```python
from build123d import *

# Parameters (mm, degrees)
BOSS_EXTRUDE1_DEPTH     = 60
SKETCH2_W               = 20
SKETCH2_H               = 25
CUT_EXTRUDE1_DEPTH      = 15
CUT_EXTRUDE2_DEPTH      = 137.47344064
CUT_EXTRUDE2_DEPTH_BACK = 137.47344064
SKETCH3_R               = 5


with BuildPart() as part:
    # Sketch1 → Boss-Extrude1 (new body)
    with BuildSketch(Plane.XY):
        Polygon((0, 0), (120, 0), (120, 43), (100, 43), (100, 15), (35, 15), (35, 25), (10, 25), (0, 20.336923418), align=None)
    extrude(amount=BOSS_EXTRUDE1_DEPTH)

    # Sketch2 → Cut-Extrude1 (cut)
    with BuildSketch(Plane(origin=(0, 43, 0), x_dir=(1, 0, 0), z_dir=(0, 1, 0))):
        with Locations((110, -30)):
            Rectangle(SKETCH2_W, SKETCH2_H)
    extrude(amount=-CUT_EXTRUDE1_DEPTH, mode=Mode.SUBTRACT)

    # Sketch3 → Cut-Extrude2 (cut, two sides: drawn at the far end of the back side and taken through both)
    with BuildSketch(Plane(origin=(0, 25, 0), x_dir=(1, 0, 0), z_dir=(0, 1, 0)).offset(-CUT_EXTRUDE2_DEPTH_BACK)):
        with Locations(Location((22.5, -40, 0), (0, 0, 180))):
            Circle(SKETCH3_R)
        with Locations(Location((22.5, -20, 0), (0, 0, 180))):
            Circle(SKETCH3_R)
    extrude(amount=CUT_EXTRUDE2_DEPTH + CUT_EXTRUDE2_DEPTH_BACK, mode=Mode.SUBTRACT)


solid = part.part
```
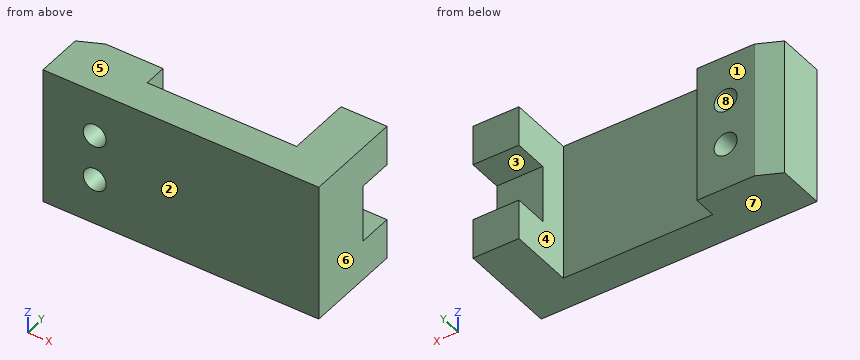
The listing builds one solid part. Answer for the finished solid, in the listing's coordinates (mm). Face numbers are marked on the shaded views. A direction names the side the tool comes from. Round coordinates to 2 decimals unless told otherwise and drop trailing zeros. Loops run counter-clockwise (first coordinate to the right, second up) from the corner with the lowest first, then second, coordinate; pieces in that order, holes last.
Q1. Section D-D, the plane y = 33.5 is taken. Determine the outline of the cut face in (x, z).
Q2. For a pull along Z with two mould halves and no side action, classify the marked faces 5, 6, 7 and 8 as released by +Z, released by -Z, zero draft, split by the parting line, or undercut.
Q3. Find the intervals of material crossed by line 1 (Z direction, x = 22.5, y = 19.5); line 2 (X direction, y = 16.5, z = 20); line 3 (X direction, y = 19, z = 56), in increasing order.
Q4. Which of the six approach directions +Z, -Z, +X, -X, +Y, -Y give full straight-line access (tool end or side, diameter ignored) to the marked faces 1, 2, 3 and 4?
Q5. Section C-C, the plane z = 20 is taken. Determine the outline of the cut face in (x, y), then the cut area to 3 significant figures.
Q6. Given pin 1 Ø2 at (x, z) = (25, 36.5) entering from -Y; pin 2 Ø10 at (x, z) = (105.5, 28) entering from +Y; pin 3 Ø8.5 at (y, z) = (31, 26) entering from -X; pin 4 Ø12 at (x, z) = (55.5, 9.5) entering from +Y, each flat-ended and moving along its own axis, determine where each tip first touches the part or whether it passes through.
Q7. Section A-A, the plane x = 22.5 is taken. Determine the outline of the cut face in (y, z).
Q8. Section B-B, the plane y = 17 is taken. Determine the outline of the cut face in (x, z), then the cut area to 3 significant figures.
Completed:
1. outline: (100, 0) - (120, 0) - (120, 17.5) - (100, 17.5) - close; (100, 42.5) - (120, 42.5) - (120, 60) - (100, 60) - close
2. face 5: released by +Z
2. face 6: zero draft
2. face 7: released by -Z
2. face 8: undercut
3. line 1: z = 0 to 15, 25 to 35, 45 to 60
3. line 2: x = 0 to 17.5, 27.5 to 35, 100 to 120
3. line 3: x = 0 to 35, 100 to 120
4. face 1: +Z, -Z, -X, +Y
4. face 2: +Z, -Z, +X, -X, -Y
4. face 3: +X, -X, +Y
4. face 4: +Z, -Z, +Y
5. outline: (0, 0) - (17.5, 0) - (17.5, 25) - (10, 25) - (0, 20.34) - close; (27.5, 0) - (120, 0) - (120, 28) - (100, 28) - (100, 15) - (35, 15) - (35, 25) - (27.5, 25) - close
5. area: 2,140 mm2
6. pin 1: stops at y = 0
6. pin 2: stops at y = 28
6. pin 3: stops at x = 100
6. pin 4: stops at y = 15
7. outline: (0, 0) - (25, 0) - (25, 15) - (0, 15) - close; (0, 25) - (25, 25) - (25, 35) - (0, 35) - close; (0, 45) - (25, 45) - (25, 60) - (0, 60) - close
8. outline: (0, 0) - (35, 0) - (35, 60) - (0, 60) - close; (100, 0) - (120, 0) - (120, 60) - (100, 60) - close; hole circle Ø10 at (22.5, 20); hole circle Ø10 at (22.5, 40)
8. area: 3,140 mm2
